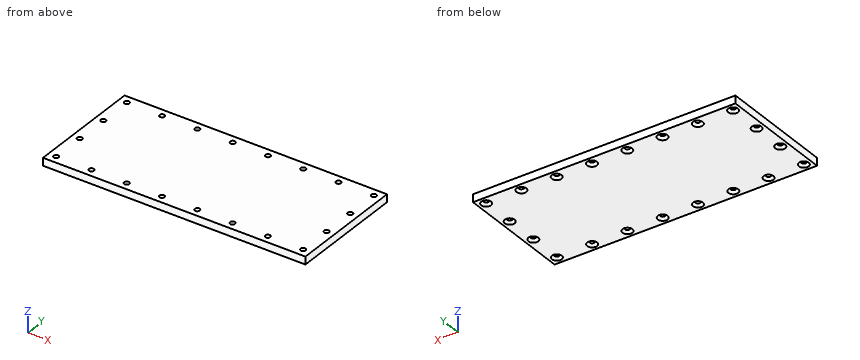
from build123d import *

# Parameters (mm, degrees)
SKETCH1_W           = 107.7
SKETCH1_H           = 47.7
SKETCH1_R           = 1.025
BOSS_EXTRUDE1_DEPTH = 3.175
CHAMFER1_SIZE       = 1


with BuildPart() as part:
    # Sketch1 → Boss-Extrude1 (new body)
    with BuildSketch(Plane.XY):
        Rectangle(SKETCH1_W, SKETCH1_H)
        with Locations((-50.675, 20.675)):
            Circle(SKETCH1_R, mode=Mode.SUBTRACT)
        with Locations((50.675, 20.675)):
            Circle(SKETCH1_R, mode=Mode.SUBTRACT)
        with Locations((-50.675, -20.675)):
            Circle(SKETCH1_R, mode=Mode.SUBTRACT)
        with Locations((50.675, -20.675)):
            Circle(SKETCH1_R, mode=Mode.SUBTRACT)
        with Locations((-7.239285714, 20.675)):
            Circle(SKETCH1_R, mode=Mode.SUBTRACT)
        with Locations((-7.239285714, -20.675)):
            Circle(SKETCH1_R, mode=Mode.SUBTRACT)
        with Locations((-36.196428571, 20.675)):
            Circle(SKETCH1_R, mode=Mode.SUBTRACT)
        with Locations((-21.717857143, 20.675)):
            Circle(SKETCH1_R, mode=Mode.SUBTRACT)
        with Locations((7.239285714, 20.675)):
            Circle(SKETCH1_R, mode=Mode.SUBTRACT)
        with Locations((21.717857143, 20.675)):
            Circle(SKETCH1_R, mode=Mode.SUBTRACT)
        with Locations((-50.675, 6.8916667)):
            Circle(SKETCH1_R, mode=Mode.SUBTRACT)
        with Locations((-50.675, -6.8916667)):
            Circle(SKETCH1_R, mode=Mode.SUBTRACT)
        with Locations((50.675, 6.8916667)):
            Circle(SKETCH1_R, mode=Mode.SUBTRACT)
        with Locations((50.675, -6.8916667)):
            Circle(SKETCH1_R, mode=Mode.SUBTRACT)
        with Locations((7.239285714, -20.675)):
            Circle(SKETCH1_R, mode=Mode.SUBTRACT)
        with Locations((21.717857143, -20.675)):
            Circle(SKETCH1_R, mode=Mode.SUBTRACT)
        with Locations((-21.717857143, -20.675)):
            Circle(SKETCH1_R, mode=Mode.SUBTRACT)
        with Locations((-36.196428571, -20.675)):
            Circle(SKETCH1_R, mode=Mode.SUBTRACT)
        with Locations((36.196428572, 20.675)):
            Circle(SKETCH1_R, mode=Mode.SUBTRACT)
        with Locations((36.196428572, -20.675)):
            Circle(SKETCH1_R, mode=Mode.SUBTRACT)
    extrude(amount=BOSS_EXTRUDE1_DEPTH)

    # Chamfer1
    chamfer1_edges = [part.edges().sort_by_distance(p)[0] for p in [
        (-51.7, 20.675, 0),
        (49.65, 20.675, 0),
        (-51.7, -20.675, 0),
        (49.65, -20.675, 0),
        (-8.264285714, 20.675, 0),
        (-8.264285714, -20.675, 0),
        (-37.221428571, 20.675, 0),
        (-22.742857143, 20.675, 0),
        (6.214285714, 20.675, 0),
        (20.692857143, 20.675, 0),
        (-51.7, 6.8916667, 0),
        (-51.7, -6.8916667, 0),
        (49.65, 6.8916667, 0),
        (49.65, -6.8916667, 0),
        (6.214285714, -20.675, 0),
        (20.692857143, -20.675, 0),
        (-22.742857143, -20.675, 0),
        (-37.221428571, -20.675, 0),
        (35.171428572, 20.675, 0),
        (35.171428572, -20.675, 0),
    ]]
    chamfer(chamfer1_edges, length=CHAMFER1_SIZE)


solid = part.part
Can you work these out from the model? Positions are in its coordinate system, mm. Give positions to 0.01 mm unless a question says otherwise; leave off trailing zeros. Answer as a JSON object with one key per item and string values.
Q1. Will these pins go through, and if not, where does the flat tip stop? P1, Ø3.5, axis at x = -21.72, y = -20.68, coming from the -Z side; P2, Ø2.5, axis at x = 36.2, y = -20.68, coming from the -Z side.
Geometry says:
{"P1": "z = 0.27", "P2": "z = 0.77"}
Q2. If I drill on L1, parallel to Y at x = 21, z = 2.1; L2, parallel to X at y = -7, z = 0.7; L3, parallel to X at y = -6, z = 1.8, over which ranges is the centre line in solid material (lowest first)?
Geometry says:
{"L1": "-23.85 to -21.41, -19.94 to 19.94, 21.41 to 23.85", "L2": "-53.85 to -52, -49.35 to 49.35, 52 to 53.85", "L3": "-53.85 to -51.18, -50.17 to 50.17, 51.18 to 53.85"}
Q3. Imagine slicing it at A-A on z = 0.5. Give the number of separate pieces and of enclosed holes in the cut face, plus the area to 3 significant figures.
Geometry says:
{"separate pieces": "1", "enclosed holes": "20", "area": "4,990 mm²"}
